Autodesk Inventor part; units mm, degrees
ref_plane "Work Plane1" through (0, 0, 125) normal (-1, 0, 0) x (0, 0, 1)
ref_plane "Work Plane2" through (590, 9, 0) normal (0, 0, -1) x (-1, 0, 0)
ref_plane "YZ Plane" through (0, 0, 0) normal (1, 0, 0) x (0, 1, 0)
sketch "Sketch1" plane through (0, 0, 0) normal (0, 1, 0) x (-1, 0, 0)
  line L0 (590, -125) -> (-590, -125)
  line L1 (-590, -125) -> (-590, 125)
  line L2 (-590, 125) -> (590, 125)
  line L3 (590, 125) -> (590, -125)
  point P0 (0, 0)
  point P1 (0, 125)
  point P2 (-590, 0)
  dimension "d0" = 250
  dimension "d1" = 1180
extrude "Extrusion1" add sketch "Sketch1" along normal blind 18
sketch "Sketch2" plane through (0, 18, 0) normal (0, 1, 0) x (1, 0, 0)
  line L0 (590, 125) -> (-590, 125)
  line L1 (-590, 125) -> (-590, -125)
  line L2 (-590, -125) -> (590, -125)
  line L3 (590, -125) -> (590, 125)
  line L4 (-590, 41.6667) -> (-572, 41.6667)
  line L5 (-572, 41.6667) -> (-572, -41.6667)
  line L6 (-572, -41.6667) -> (-590, -41.6667)
  line L7 (-590, -41.6667) -> (-590, 41.6667)
  line L8 (-590, 125) -> (-590, -125)
  point P0 (0, 0)
  point P1 (-572, 0)
  point P2 (-590, 0)
  point P3 (-590, 0)
  point P4 (-590, 0)
  dimension "d4" = 18
  dimension "d5" = 83.3333
extrude "Extrusion2" cut sketch "Sketch2" against normal blind 9 contours L4 L5 L6 L1
ref_plane "Work Plane1" through (0, 0, 125) normal (-1, 0, 0) x (0, 0, 1)
mirror "Mirror1" about plane through (0, 0, 125) normal (-1, 0, 0) of "Extrusion2"
sketch "Sketch3" plane through (0, 18, 0) normal (0, 1, 0) x (1, 0, 0)
  line L0 (590, -41.6667) -> (572, -41.6667)
  line L1 (572, -41.6667) -> (572, 41.6667)
  line L2 (572, 41.6667) -> (590, 41.6667)
  line L3 (590, 41.6667) -> (590, 125)
  line L4 (590, 125) -> (-590, 125)
  line L5 (-590, 125) -> (-590, 41.6667)
  line L6 (-590, 41.6667) -> (-572, 41.6667)
  line L7 (-572, 41.6667) -> (-572, -41.6667)
  line L8 (-572, -41.6667) -> (-590, -41.6667)
  line L9 (-590, -41.6667) -> (-590, -125)
  line L10 (-590, -125) -> (590, -125)
  line L11 (590, -125) -> (590, -41.6667)
  line L12 (-336.7778, 41.6667) -> (-318.7778, 41.6667)
  line L13 (-318.7778, 41.6667) -> (-318.7778, -41.6667)
  line L14 (-318.7778, -41.6667) -> (-336.7778, -41.6667)
  line L15 (-336.7778, -41.6667) -> (-336.7778, 41.6667)
  line L16 (-318.7778, 41.6667) -> (-327.7778, 41.6667) construction
  point P0 (0, 0)
  point P1 (-318.7778, 0)
  point P2 (-572, 0)
  point P3 (-323.2778, 41.6667)
  point P4 (-327.7778, 41.6667)
  dimension "d9" = 18
  dimension "d10" = 83.3333
  dimension "d11" = 83.3333
  dimension "d15" = 9
  dimension "d16" = 262.2222
extrude "Extrusion3" cut sketch "Sketch3" against normal blind 9 contours L12 L13 L14 L15
mirror "Mirror2" about plane through (0, 0, 125) normal (-1, 0, 0) of "Extrusion3"
sketch "Sketch4" plane through (0, 18, 0) normal (0, 1, 0) x (1, 0, 0)
  line L0 (336.7778, 41.6667) -> (336.7778, -41.6667)
  line L1 (336.7778, -41.6667) -> (318.7778, -41.6667)
  line L2 (318.7778, -41.6667) -> (318.7778, 41.6667)
  line L3 (318.7778, 41.6667) -> (336.7778, 41.6667)
  line L4 (-336.7778, -41.6667) -> (-336.7778, 41.6667)
  line L5 (-336.7778, 41.6667) -> (-318.7778, 41.6667)
  line L6 (-318.7778, 41.6667) -> (-318.7778, -41.6667)
  line L7 (-318.7778, -41.6667) -> (-336.7778, -41.6667)
  line L8 (590, -41.6667) -> (572, -41.6667)
  line L9 (572, -41.6667) -> (572, 41.6667)
  line L10 (572, 41.6667) -> (590, 41.6667)
  line L11 (590, 41.6667) -> (590, 125)
  line L12 (590, 125) -> (-590, 125)
  line L13 (-590, 125) -> (-590, 41.6667)
  line L14 (-590, 41.6667) -> (-572, 41.6667)
  line L15 (-572, 41.6667) -> (-572, -41.6667)
  line L16 (-572, -41.6667) -> (-590, -41.6667)
  line L17 (-590, -41.6667) -> (-590, -125)
  line L18 (-590, -125) -> (590, -125)
  line L19 (590, -125) -> (590, -41.6667)
  point P0 (0, 0)
  point P1 (572, -38.4917)
  dimension "d17" = 3.175
hole "Hole1" at (572, 18, 38.4917) direction (0, -1, 0) diameter 6.35 depth 9 tip angle 118
ref_plane "Work Plane2" through (590, 9, 0) normal (0, 0, -1) x (-1, 0, 0)
mirror "Mirror3" about plane through (590, 9, 0) normal (0, 0, -1) of "Hole1"
mirror "Mirror4" about plane through (0, 0, 125) normal (-1, 0, 0) of "Hole1", "Mirror3"
sketch "Sketch5" plane through (318.7778, 9, -41.6667) normal (0, 1, 0) x (1, 0, 0)
  line L0 (18, 0) -> (18, -83.3333)
  line L1 (18, -83.3333) -> (0, -83.3333)
  line L2 (0, -83.3333) -> (0, 0)
  line L3 (0, 0) -> (18, 0)
  line L4 (-655.5556, -83.3333) -> (-655.5556, 0)
  line L5 (-655.5556, 0) -> (-637.5556, 0)
  line L6 (-637.5556, 0) -> (-637.5556, -83.3333)
  line L7 (-637.5556, -83.3333) -> (-655.5556, -83.3333)
  arc A0 (-890.7778, -6.35) -> (-890.7778, 0) centre (-890.7778, -3.175) ccw
  line L8 (-890.7778, -6.35) -> (-890.7778, -76.9833)
  arc A1 (-890.7778, -83.3333) -> (-890.7778, -76.9833) centre (-890.7778, -80.1583) ccw
  line L9 (-890.7778, -83.3333) -> (-908.7778, -83.3333)
  line L10 (-908.7778, -83.3333) -> (-908.7778, -166.6667)
  line L11 (-908.7778, -166.6667) -> (271.2222, -166.6667)
  line L12 (271.2222, -166.6667) -> (271.2222, -83.3333)
  line L13 (271.2222, -83.3333) -> (253.2222, -83.3333)
  arc A2 (253.2222, -76.9833) -> (253.2222, -83.3333) centre (253.2222, -80.1583) ccw
  line L14 (253.2222, -76.9833) -> (253.2222, -6.35)
  arc A3 (253.2222, 0) -> (253.2222, -6.35) centre (253.2222, -3.175) ccw
  line L15 (253.2222, 0) -> (271.2222, 0)
  line L16 (271.2222, 0) -> (271.2222, 83.3333)
  line L17 (271.2222, 83.3333) -> (-908.7778, 83.3333)
  line L18 (-908.7778, 83.3333) -> (-908.7778, 0)
  line L19 (-908.7778, 0) -> (-890.7778, 0)
  point P0 (-318.7778, -41.6667)
  point P1 (14.825, -83.3333)
  point P2 (3.175, -83.3333)
  dimension "d25" = 3.175
  dimension "d26" = 3.175
hole "Hole2" at (333.6028, 9, 41.6667) at (321.9528, 9, 41.6667) direction (0, 1, 0) diameter 6.35 depth 9 tip angle 118
mirror "Mirror5" about plane through (590, 9, 0) normal (0, 0, -1) of "Hole2"
mirror "Mirror6" about plane through (0, 0, 125) normal (-1, 0, 0) of "Hole2", "Mirror5"
sketch "Sketch7" plane through (0, 18, 0) normal (0, 1, 0) x (1, 0, 0)
  arc A0 (336.7778, 41.6667) -> (330.4278, 41.6667) centre (333.6028, 41.6667) ccw
  line L0 (336.7778, 41.6667) -> (336.7778, -41.6667)
  arc A1 (330.4278, -41.6667) -> (336.7778, -41.6667) centre (333.6028, -41.6667) ccw
  line L1 (330.4278, -41.6667) -> (325.1278, -41.6667)
  arc A2 (318.7778, -41.6667) -> (325.1278, -41.6667) centre (321.9528, -41.6667) ccw
  line L2 (318.7778, -41.6667) -> (318.7778, 41.6667)
  arc A3 (325.1278, 41.6667) -> (318.7778, 41.6667) centre (321.9528, 41.6667) ccw
  line L3 (325.1278, 41.6667) -> (330.4278, 41.6667)
  arc A4 (-572, 35.3167) -> (-572, 41.6667) centre (-572, 38.4917) ccw
  line L4 (-572, 35.3167) -> (-572, -35.3167)
  arc A5 (-572, -41.6667) -> (-572, -35.3167) centre (-572, -38.4917) ccw
  line L5 (-572, -41.6667) -> (-590, -41.6667)
  line L6 (-590, -41.6667) -> (-590, -125)
  line L7 (-590, -125) -> (590, -125)
  line L8 (590, -125) -> (590, -41.6667)
  line L9 (590, -41.6667) -> (572, -41.6667)
  arc A6 (572, -35.3167) -> (572, -41.6667) centre (572, -38.4917) ccw
  line L10 (572, -35.3167) -> (572, 35.3167)
  arc A7 (572, 41.6667) -> (572, 35.3167) centre (572, 38.4917) ccw
  line L11 (572, 41.6667) -> (590, 41.6667)
  line L12 (590, 41.6667) -> (590, 125)
  line L13 (590, 125) -> (-590, 125)
  line L14 (-590, 125) -> (-590, 41.6667)
  line L15 (-590, 41.6667) -> (-572, 41.6667)
  arc A8 (-330.4278, 41.6667) -> (-336.7778, 41.6667) centre (-333.6028, 41.6667) ccw
  line L16 (-330.4278, 41.6667) -> (-325.1278, 41.6667)
  arc A9 (-318.7778, 41.6667) -> (-325.1278, 41.6667) centre (-321.9528, 41.6667) ccw
  line L17 (-318.7778, 41.6667) -> (-318.7778, -41.6667)
  arc A10 (-325.1278, -41.6667) -> (-318.7778, -41.6667) centre (-321.9528, -41.6667) ccw
  line L18 (-325.1278, -41.6667) -> (-330.4278, -41.6667)
  arc A11 (-336.7778, -41.6667) -> (-330.4278, -41.6667) centre (-333.6028, -41.6667) ccw
  line L19 (-336.7778, -41.6667) -> (-336.7778, 41.6667)
  point P0 (0, 0)
  point P1 (581, -83.3333)
  point P2 (581, 83.3333)
  point P3 (590, 83.3333)
  point P4 (590, -83.3333)
  dimension "d34" = 9
  dimension "d35" = 9
hole "Hole3" at (581, 18, 83.3333) at (581, 18, -83.3333) direction (0, -1, 0) diameter 6.35 end through all
mirror "Mirror7" about plane through (0, 0, 125) normal (-1, 0, 0) of "Hole3"
equation "\"d0\" = shelfWidth"
equation "\"d1\" = shelfLength"
equation "\"d2\" = plyThickness"
equation "\"d4\" = plyThickness"
equation "\"d5\" = 0.333333 * shelfWidth"
equation "\"d7\" = 0.5 * plyThickness"
equation "\"d9\" = plyThickness"
equation "\"d10\" = 0.333333 * shelfWidth"
equation "\"d15\" = 0.5 * plyThickness"
equation "\"d16\" = 0.222222 * shelfLength"
equation "\"d13\" = 0.5 * plyThickness"
equation "\"d18\" = millDiameter"
equation "\"d23\" = 0.5 * plyThickness"
equation "\"d27\" = millDiameter"
equation "\"d32\" = 0.5 * plyThickness"
equation "\"d36\" = millDiameter"
equation "\"d41\" = 0.5 * plyThickness"
equation "\"plyThickness\" = 18"
equation "\"legHeight\" = 702"
equation "\"millDiameter\" = 6.35"
equation "\"legTopTabHeight\" = 18"
equation "\"legTopSlotDepth\" = 49"
equation "\"shelfLength\" = 1180"
equation "\"shelfWidth\" = 250"
properties part number "shelfTop"
Could you check a few things on this model? Use its own coordinates, in mm. Coordinates: 2 decimals unless noted, no trailing zeros. Loops run counter-clockwise (first coordinate to the right, second up) from the corner with the lowest first, then second, coordinate; pieces in that order, holes last.
1) Will these pins go through, and if not, where does the flat tip stop? pin 1 Ø7 at (y, z) = (15, -19.5) entering from -X; pin 2 Ø2.5 at (y, z) = (11.5, 0.5) entering from +X.
Reported:
pin 1: stops at x = -572
pin 2: stops at x = 572
2) Please list where these lines run through material, in increasing order: line 1 along X through (y, z) = (12.25, 25); line 2 along X through (y, z) = (7.75, 82.5); line 3 along Z through (x, y) = (581, 10.75).
Reported:
line 1: x = -572 to -336.78, -318.78 to 318.78, 336.78 to 572
line 2: x = -590 to -584.06, -577.94 to 577.94, 584.06 to 590
line 3: z = -125 to -86.51, -80.16 to -41.67, 41.67 to 80.16, 86.51 to 125
3) Imagine slicing it at A-A (z = 25). List the corners of the cut face in (x, y) for me, and give its area (3 significant figures).
Reported:
outline: (-590, 0) - (590, 0) - (590, 9) - (572, 9) - (572, 18) - (336.78, 18) - (336.78, 9) - (318.78, 9) - (318.78, 18) - (-318.78, 18) - (-318.78, 9) - (-336.78, 9) - (-336.78, 18) - (-572, 18) - (-572, 9) - (-590, 9) - close
area: 20,600 mm2
